CAD build for the part. Positions are in the model's coordinates, mm. Face numbers are marked on the shaded views. Give positions to 0.01 mm unless a question says otherwise; leave off trailing zeros. Loops run counter-clockwise (first coordinate to the right, second up) from the corner with the lowest first, then second, coordinate; pieces in that order, holes last. Notation, with made-up numbers: M -8,32.25 L 23,32.25 A23 ccw 23,66.25 Z; hole C 18.5,-22.5 d7. An arc over 180 degrees is marked long. Answer as CSV lines item,"result".
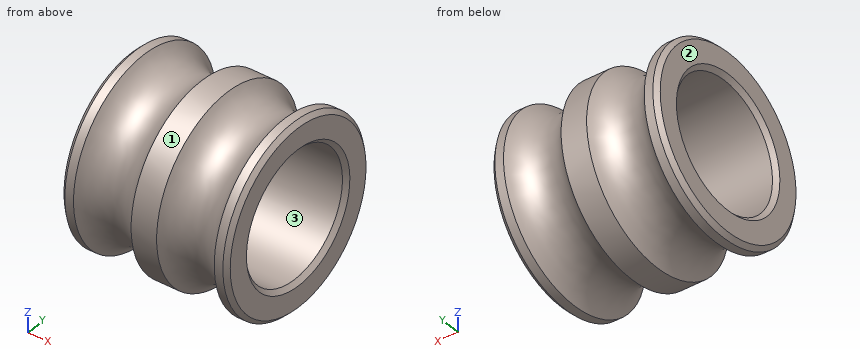
```python
from build123d import *

# Parameters (mm, degrees)
F1_W    = 40
F1_H    = 7
F3_SIZE = 1
F0_R    = 8


with BuildPart() as f2:
    # F1 (on Front) → F2 (revolve)
    with BuildSketch(Plane.XZ):
        with Locations((0, 18.5)):
            Rectangle(F1_W, F1_H)
    revolve(axis=Axis((0, 0, 0), (1, 0, 0)))

    # F3
    f3_edges = [f2.edges().sort_by_distance(p)[0] for p in [
        (-20, 0, -22),
        (-20, 0, -15),
        (20, 0, -22),
        (20, 0, -15),
    ]]
    chamfer(f3_edges, length=F3_SIZE)

    # F0 (on Front) → F4 (revolve, cut)
    with BuildSketch(Plane.XZ):
        with Locations((-10, 26)):
            Circle(F0_R)
        with Locations((10, 26)):
            Circle(F0_R)
    revolve(axis=Axis((0, 0, 0), (1, 0, 0)), mode=Mode.SUBTRACT)


solid = f2.part
```
Q1. Cut at D-D (y = -18). Give the number of separate pieces and of enclosed holes in the cut face, and give its area (3 significant figures).
Solution:
separate pieces,"3"
enclosed holes,"0"
area,"621 mm²"
Q2. Pin check, flat tips, straight feed: P1, Ø5, axis at x = -2, z = 1.5, coming from the -Y side; P2, Ø1.5, axis at x = 12.5, y = -16, coming from the +Z side; P3, Ø12, axis at x = -7.5, z = -4, coming from the +Y side. Stop position of each tip, or through.
Solution:
P1,"stops at y = -22"
P2,"stops at z = 10.39"
P3,"stops at y = 22"
Q3. Cut at A-A (y = 0). Write the cut outline in (x, z).
Solution:
outline,"M -20,-21 L -19,-22 L -16.93,-22 A8 cw -3.07,-22 L 3.07,-22 A8 cw 16.93,-22 L 19,-22 L 20,-21 L 20,-16 L 19,-15 L -19,-15 L -20,-16 Z; M -20,16 L -19,15 L 19,15 L 20,16 L 20,21 L 19,22 L 16.93,22 A8 cw 3.07,22 L -3.07,22 A8 cw -16.93,22 L -19,22 L -20,21 Z"
Q4. Wall check: line 1 (Y direction, x = 0, z = 0); line 2 (X direction, y = 1.5, z = -19). Give the ranges that are in metal, low to high. Write a range as [from, to].
Solution:
line 1,"y = [-22, -15], [15, 22]"
line 2,"x = [-20, -13.98], [-6.02, 6.02], [13.98, 20]"
Q5. Cut at C-C (x = 5). Write the cut outline in (y, z) (3 decimals), and give its area (3 significant figures).
Solution:
outline,"C 0,0 d39.51; hole C 0,0 d30"
area,"519 mm²"
Q6. Mould opens along Z. For the marked faces 1, 2 and 3 say: released by +Z, released by -Z, zero draft, split by the parting line, or undercut.
Solution:
face 1,"split by the parting line"
face 2,"zero draft"
face 3,"undercut"
